Geometry: final body of the model. Coordinates: model frame, mm. Coordinates: 2 decimals unless noted, no trailing zeros. Order: outer loops, then holes, each group sorted by start corner. A loop starts at its lowest first (then second) coordinate and runs counter-clockwise, first axis right, second up. Notation, with made-up numbers: (60.5, -29.75) - (106.5, -29.75) arc R24 ccw to (106.5, -7.75) - close; hole circle Ø6 at (25.5, -3.75). An arc over 180 degrees is marked (long way). Use a Markdown table: item, result. Add a question column.
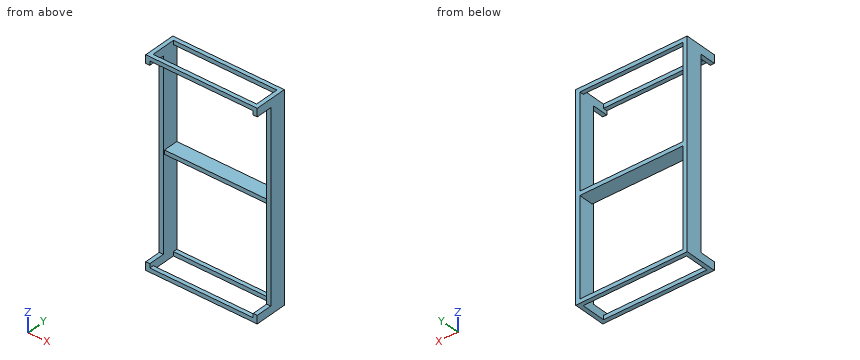
```python
from build123d import *

# Parameters (mm, degrees)
SKETCH1_W           = 550
SKETCH1_H           = 160
SKETCH1_W_2         = 510
SKETCH1_H_2         = 120
BOSS_EXTRUDE1_DEPTH = 1000
SKETCH2_W           = 920
SKETCH2_H           = 80
CUT_EXTRUDE1_DEPTH  = 1000
SKETCH3_W           = 510
SKETCH3_H           = 960
CUT_EXTRUDE3_DEPTH  = 1000
SKETCH4_W           = 550
SKETCH4_H           = 20
BOSS_EXTRUDE2_DEPTH = 73


with BuildPart() as part:
    # Sketch1 → Boss-Extrude1 (new body)
    with BuildSketch(Plane.XY):
        with Locations((255, 60)):
            Rectangle(SKETCH1_W, SKETCH1_H)
        with Locations((255, 60)):
            Rectangle(SKETCH1_W_2, SKETCH1_H_2, mode=Mode.SUBTRACT)
    extrude(amount=BOSS_EXTRUDE1_DEPTH)

    # Sketch2 → Cut-Extrude1 (cut)
    with BuildSketch(Plane.ZY.offset(20)):
        with Locations((500, 20)):
            Rectangle(SKETCH2_W, SKETCH2_H)
    extrude(amount=-CUT_EXTRUDE1_DEPTH, mode=Mode.SUBTRACT)

    # Sketch3 → Cut-Extrude3 (cut)
    with BuildSketch(Plane(origin=(0, 140, 0), x_dir=(1, 0, 0), z_dir=(0, 1, 0))):
        with Locations((255, -500)):
            Rectangle(SKETCH3_W, SKETCH3_H)
    extrude(amount=-CUT_EXTRUDE3_DEPTH, mode=Mode.SUBTRACT)

    # Sketch4 → Boss-Extrude2 (add)
    with BuildSketch(Plane(origin=(0, 140, 0), x_dir=(1, 0, 0), z_dir=(0, 1, 0))):
        with Locations((255, -510)):
            Rectangle(SKETCH4_W, SKETCH4_H)
    extrude(amount=-BOSS_EXTRUDE2_DEPTH)


solid = part.part
```
1) Pin query (flat end, axial travel): pin 1 (10 mm diameter, centred on x = 241, z = 513, fed in from -Y); pin 2 (22 mm diameter, centred on x = 520.5, z = 306.5, fed in from -Y). Return the tip coordinate at first contact, or that it passes through.
2) Section A-A (y = 19). Return loops of the section in (x, z), then the cut area to 3 significant figures.
3) Section C-C (x = 345.5). Return loops of the section in (y, z).
4) Ray query, line 1 along Z through (x, y) = (299, 132.5); line 2 along X through (y, z) = (116.5, 856.5); line 3 along Z through (x, y) = (91.5, 91). Return the intervals inside material, ascending.
5) Section B-B (z = 433). Return loops of the section in (x, y), then the cut area to 3 significant figures.
Values follow:
| question | item | result |
|---|---|---|
| 1 | pin 1 | stops at y = 67 |
| 1 | pin 2 | stops at y = 60 |
| 2 | outline | (-20, 0) - (0, 0) - (0, 40) - (-20, 40) - close; (-20, 960) - (0, 960) - (0, 1000) - (-20, 1000) - close; (510, 0) - (530, 0) - (530, 40) - (510, 40) - close; (510, 960) - (530, 960) - (530, 1000) - (510, 1000) - close |
| 2 | area | 3,200 mm² |
| 3 | outline | (-20, 0) - (0, 0) - (0, 20) - (-20, 20) - close; (-20, 980) - (0, 980) - (0, 1000) - (-20, 1000) - close; (67, 500) - (140, 500) - (140, 520) - (67, 520) - close; (120, 0) - (140, 0) - (140, 20) - (120, 20) - close; (120, 980) - (140, 980) - (140, 1000) - (120, 1000) - close |
| 4 | line 1 | z = 0 to 20, 500 to 520, 980 to 1000 |
| 4 | line 2 | x = -20 to 0, 510 to 530 |
| 4 | line 3 | z = 500 to 520 |
| 5 | outline | (-20, 60) - (0, 60) - (0, 140) - (-20, 140) - close; (510, 60) - (530, 60) - (530, 140) - (510, 140) - close |
| 5 | area | 3,200 mm² |
